Autodesk Fusion 360 part; units mm, degrees
sketch "Sketch1" plane through (0, 0, 0) normal (0, 0, 1) x (1, 0, 0)
  circle A0 centre (0, 0) radius 4
  circle A1 centre (0, 0) radius 3
  circle A2 centre (0, 0) radius 6.55
  dimension "d1" = 8
  dimension "d2" = 6
  dimension "d3" = 13.1
extrude "Extrude1" add sketch "Sketch1" along normal blind 2.7 makes body 1 at (6.5419, -0.3265, 1.8) makes body 2 at (2.9963, -0.1495, 1.8)
extrude "Extrude2" add 1 faces at (-1.1591, 0.5829, 2.7) along direction (0, 0, 1) blind 1.3 on bodies 2 bodies 2
extrude "Extrude3" add sketch "Sketch1" along normal blind 10.7 contours A0 bodies 1 2
sketch "Sketch2" plane through (0, 0, 0) normal (0, 0, -1) x (1, 0, 0)
  circle A0 centre (0, 0) radius 6.55
  line L0 (-2, 0) -> (2, 0) construction
  line L1 (1, -1.7321) -> (-1, 1.7321) construction
  line L2 (1, 1.7321) -> (-1, -1.7321) construction
  line L3 (-2, -2.5) -> (-2, 2.5) construction
  line L4 (-2, 2.5) -> (2, 2.5) construction
  line L5 (2, 2.5) -> (2, -2.5) construction
  line L6 (2, -2.5) -> (-2, -2.5) construction
  line L7 (-1, -1.7321) -> (-2, -1.1547) construction
  line L8 (-1, 1.7321) -> (-2, 1.1547) construction
  line L9 (-2, -1.1547) -> (-2, 1.1547)
  line L10 (1, -1.7321) -> (2, -1.1547) construction
  line L11 (1, 1.7321) -> (2, 1.1547) construction
  line L12 (-2, -1.1547) -> (0, -2.3094)
  line L13 (0, -2.3094) -> (2, -1.1547)
  line L14 (2, 1.1547) -> (0, 2.3094)
  line L15 (0, 2.3094) -> (-2, 1.1547)
  line L16 (2, -1.1547) -> (2, 1.1547)
  dimension "d10" = 4
  dimension "d12" = 360
extrude "Extrude4" cut sketch "Sketch2" against normal blind 2 contours L9 L12 L13 L14 L15 L16 bodies 1
chamfer "Chamfer1" distance 0.5 distance2 1.9 6 edges at (-1, 1.7321, 2) (1, 1.7321, 2) (2, 0, 2) (1, -1.7321, 2) (-2, 0, 2) (-1, -1.7321, 2) measured on face at (-1.3333, 1.5396, 0.6667) measured on face at (0.6667, 1.9245, 0.6667) measured on face at (2, 0.3849, 0.6667) measured on face at (1.3333, -1.5396, 0.6667) measured on face at (-2, 0.3849, 0.6667) measured on face at (-0.6667, -1.9245, 0.6667) on bodies 1
chamfer "Chamfer2" distance 0.5 distance2 0.2 6 edges at (2, 0, 0) (1, -1.7321, 0) (-1, -1.7321, 0) (-2, 0, 0) (-1, 1.7321, 0) (1, 1.7321, 0) measured on face at (1.7583, -3.0455, 0) measured on face at (1.7583, -3.0455, 0) measured on face at (1.7583, -3.0455, 0) measured on face at (1.7583, -3.0455, 0) measured on face at (1.7583, -3.0455, 0) measured on face at (1.7583, -3.0455, 0) on bodies 1
chamfer "Chamfer3" distance 1 distance2 2 1 edges at (-6.1067, -2.3686, 0) measured on face at (6.5419, -0.3265, 1.8) on bodies 1
fillet "Fillet1" radius 0.75 1 edges at (-6.1067, -2.3686, 2.7) on bodies 1
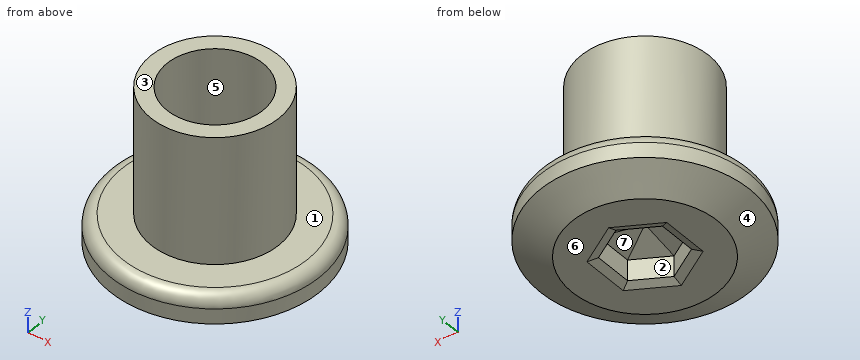
Design review of the part built by this model. Coordinates are the model's own, in mm. Face numbers are marked on the shaded views. A direction names the side the tool comes from. Round coordinates to 2 decimals unless told otherwise and drop trailing zeros. Write each loop counter-clockwise with the first axis right and the second up, starting at its lowest first coordinate (ties: lowest second). Pieces come first, ordered by that corner, then holes.
Item 1: For the marked faces 1, 2 and 3, list the 3-axis set-ups (+Z, -Z, +X, -X, +Y, -Y) from which the entire face can be reached by the end or side of a thin tool; tool diameter is ignored.
Item 2: Consider section A-A on z = 8.5. Give the boundary of the cut face in (x, y).
Item 3: Wall thickness on L1, parallel to Y at x = 0, z = 5.75; L2, parallel to Y at x = 2.75, z = 9.5; L3, parallel to X at y = 2.5, z = 8: over which ranges is each line inside the solid? List them lowest first.
Item 4: Draft analysis for pull direction X (two halves, no side actions). For the marked faces 4, 5, 6 and 7, state which applies: released by +X, released by -X, zero draft, split by the parting line, or undercut.
Item 5: For pin 1 Ø1 at (x, z) = (-5, 7) entering from +Y; pin 2 Ø2 at (x, z) = (-1.5, 5.5) entering from +Y; pin 3 Ø2 at (x, z) = (3.5, 2.5) entering from -Y; pin 4 Ø3 at (x, y) = (0.5, -1) entering from +Z, all flat-tipped, find the tip position at first contact; note any pin that passes through.
Check values:
1. face 1: +Z
1. face 2: -Z
1. face 3: +Z, +X, -X, +Y, -Y
2. outline: circle Ø8 at (0, 0); hole circle Ø6 at (0, 0)
3. L1: y = -4 to -3, 3 to 4
3. L2: y = -2.9 to -1.2, 1.2 to 2.9
3. L3: x = -3.12 to -1.66, 1.66 to 3.12
4. face 4: split by the parting line
4. face 5: undercut
4. face 6: zero draft
4. face 7: undercut
5. pin 1: passes through
5. pin 2: stops at y = 3.97
5. pin 3: stops at y = -6
5. pin 4: stops at z = 4
